Check sheet for the modelled part. Datum: model origin and axes. Units: mm. A direction names the side the tool comes from. Give positions to 0.01 mm unless a question says otherwise; leave off trailing zeros. Write each loop counter-clockwise with the first axis right and the second up, starting at its lowest first coordinate (ties: lowest second). Pieces come first, ordered by that corner, then holes. Notation, with made-up numbers: (72.5, 57) -> (83.5, 57) arc R21 cw to (83.5, 74) -> close; hole circle Ø6 at (67, 55). An arc over 180 degrees is marked (long way). Use a Markdown table: item, result. Add a question column.
1. Cross-section at A-A (x = -2.25). Enter the section's corners in (y, z).
2. Cross-section at B-B (y = -7.5). Enter the section's corners in (x, z).
3. Scan lines: probe 1 along Y at (x, z) = (0, 13); probe 2 along X at (y, z) = (-8.75, -19); probe 3 along X at (y, z) = (-1.5, 19.5). Record each from-to range of solid material in increasing order. Write a range as [from, to].
4. Release check for a two-part mould opening along Y. For faces 1 (the flat face through (0.754, 13.708, 0.35)), 2 (the flat face through (-12.804, 4.953, 0.35)), 3 (the flat face through (-5, 9, -25)), 4 (the flat face through (-3.537, -13.302, 0.35)) record: released by +Y, released by -Y, zero draft, split by the parting line, or undercut.
5. Set-up check for faces 5 (the cylindrical face through (-12.344, 1.969, 0.35)), 6 (the flat face through (7.474, 11.558, 0.35)), 7 (the cylindrical face through (8.85, 8.83, 0.35)): record each of +Z, -Z, +X, -X, +Y, -Y from which the full face is reachable in a straight line by a thin tool's end or side.
6. Gauge pin test, flat ends, axial feed: P1, Ø10, axis at y = 9, z = 4.5, coming from the -X side; P2, Ø3, axis at x = -12, z = 10.5, coming from the -Y side; P3, Ø1, axis at y = 8, z = 19.5, coming from the -X side. Record the tip position at first contact, or that the pin passes through.
from build123d import *

# Parameters (mm, degrees)
SKETCH1_R           = 10
BOSS_EXTRUDE1_DEPTH = 25


with BuildPart() as part:
    # Sketch1 → Boss-Extrude1 (new, symmetric)
    with BuildSketch(Plane.XY):
        with BuildLine():
            Line((-0.5, 14.991664351), (-1, 12.459935794))
            ThreePointArc((-1, 12.459935794), (-1.955430813, 12.346104257), (-2.899275393, 12.159120124))
            Line((-2.899275393, 12.159120124), (-4.1571508, 14.412428568))
            ThreePointArc((-4.1571508, 14.412428568), (-4.635254916, 14.265847744), (-5.108207316, 14.103411574))
            Line((-5.108207316, 14.103411574), (-4.801388426, 11.541086135))
            ThreePointArc((-4.801388426, 11.541086135), (-5.674881247, 11.137581552), (-6.51474951, 10.668085059))
            Line((-6.51474951, 10.668085059), (-8.407370715, 12.42240386))
            ThreePointArc((-8.407370715, 12.42240386), (-8.816778784, 12.135254916), (-9.21638771, 11.834618607))
            Line((-9.21638771, 11.834618607), (-8.132783499, 9.492514554))
            ThreePointArc((-8.132783499, 9.492514554), (-8.838834765, 8.838834765), (-9.492514554, 8.132783499))
            Line((-9.492514554, 8.132783499), (-11.834618607, 9.21638771))
            ThreePointArc((-11.834618607, 9.21638771), (-12.135254916, 8.816778784), (-12.42240386, 8.407370715))
            Line((-12.42240386, 8.407370715), (-10.668085059, 6.51474951))
            ThreePointArc((-10.668085059, 6.51474951), (-11.137581552, 5.674881247), (-11.541086135, 4.801388426))
            Line((-11.541086135, 4.801388426), (-14.103411574, 5.108207316))
            ThreePointArc((-14.103411574, 5.108207316), (-14.265847744, 4.635254916), (-14.412428568, 4.1571508))
            Line((-14.412428568, 4.1571508), (-12.159120124, 2.899275393))
            ThreePointArc((-12.159120124, 2.899275393), (-12.346104257, 1.955430813), (-12.459935794, 1))
            Line((-12.459935794, 1), (-14.991664351, 0.5))
            ThreePointArc((-14.991664351, 0.5), (-15, 0), (-14.991664351, -0.5))
            Line((-14.991664351, -0.5), (-12.459935794, -1))
            ThreePointArc((-12.459935794, -1), (-12.346104257, -1.955430813), (-12.159120124, -2.899275393))
            Line((-12.159120124, -2.899275393), (-14.412428568, -4.1571508))
            ThreePointArc((-14.412428568, -4.1571508), (-14.265847744, -4.635254916), (-14.103411574, -5.108207316))
            Line((-14.103411574, -5.108207316), (-11.541086135, -4.801388426))
            ThreePointArc((-11.541086135, -4.801388426), (-11.137581552, -5.674881247), (-10.668085059, -6.51474951))
            Line((-10.668085059, -6.51474951), (-12.42240386, -8.407370715))
            ThreePointArc((-12.42240386, -8.407370715), (-12.135254916, -8.816778784), (-11.834618607, -9.21638771))
            Line((-11.834618607, -9.21638771), (-9.492514554, -8.132783499))
            ThreePointArc((-9.492514554, -8.132783499), (-8.838834765, -8.838834765), (-8.132783499, -9.492514554))
            Line((-8.132783499, -9.492514554), (-9.21638771, -11.834618607))
            ThreePointArc((-9.21638771, -11.834618607), (-8.816778784, -12.135254916), (-8.407370715, -12.42240386))
            Line((-8.407370715, -12.42240386), (-6.51474951, -10.668085059))
            ThreePointArc((-6.51474951, -10.668085059), (-5.674881247, -11.137581552), (-4.801388426, -11.541086135))
            Line((-4.801388426, -11.541086135), (-5.108207316, -14.103411574))
            ThreePointArc((-5.108207316, -14.103411574), (-4.635254916, -14.265847744), (-4.1571508, -14.412428568))
            Line((-4.1571508, -14.412428568), (-2.899275393, -12.159120124))
            ThreePointArc((-2.899275393, -12.159120124), (-1.955430813, -12.346104257), (-1, -12.459935794))
            Line((-1, -12.459935794), (-0.5, -14.991664351))
            ThreePointArc((-0.5, -14.991664351), (0, -15), (0.5, -14.991664351))
            Line((0.5, -14.991664351), (1, -12.459935794))
            ThreePointArc((1, -12.459935794), (1.955430813, -12.346104257), (2.899275393, -12.159120124))
            Line((2.899275393, -12.159120124), (4.1571508, -14.412428568))
            ThreePointArc((4.1571508, -14.412428568), (4.635254916, -14.265847744), (5.108207316, -14.103411574))
            Line((5.108207316, -14.103411574), (4.801388426, -11.541086135))
            ThreePointArc((4.801388426, -11.541086135), (5.674881247, -11.137581552), (6.51474951, -10.668085059))
            Line((6.51474951, -10.668085059), (8.407370715, -12.42240386))
            ThreePointArc((8.407370715, -12.42240386), (8.816778784, -12.135254916), (9.21638771, -11.834618607))
            Line((9.21638771, -11.834618607), (8.132783499, -9.492514554))
            ThreePointArc((8.132783499, -9.492514554), (8.838834765, -8.838834765), (9.492514554, -8.132783499))
            Line((9.492514554, -8.132783499), (11.834618607, -9.21638771))
            ThreePointArc((11.834618607, -9.21638771), (12.135254916, -8.816778784), (12.42240386, -8.407370715))
            Line((12.42240386, -8.407370715), (10.668085059, -6.51474951))
            ThreePointArc((10.668085059, -6.51474951), (11.137581552, -5.674881247), (11.541086135, -4.801388426))
            Line((11.541086135, -4.801388426), (14.103411574, -5.108207316))
            ThreePointArc((14.103411574, -5.108207316), (14.265847744, -4.635254916), (14.412428568, -4.1571508))
            Line((14.412428568, -4.1571508), (12.159120124, -2.899275393))
            ThreePointArc((12.159120124, -2.899275393), (12.346104257, -1.955430813), (12.459935794, -1))
            Line((12.459935794, -1), (14.991664351, -0.5))
            ThreePointArc((14.991664351, -0.5), (15, 0), (14.991664351, 0.5))
            Line((14.991664351, 0.5), (12.459935794, 1))
            ThreePointArc((12.459935794, 1), (12.346104257, 1.955430813), (12.159120124, 2.899275393))
            Line((12.159120124, 2.899275393), (14.412428568, 4.1571508))
            ThreePointArc((14.412428568, 4.1571508), (14.265847744, 4.635254916), (14.103411574, 5.108207316))
            Line((14.103411574, 5.108207316), (11.541086135, 4.801388426))
            ThreePointArc((11.541086135, 4.801388426), (11.137581552, 5.674881247), (10.668085059, 6.51474951))
            Line((10.668085059, 6.51474951), (12.42240386, 8.407370715))
            ThreePointArc((12.42240386, 8.407370715), (12.135254916, 8.816778784), (11.834618607, 9.21638771))
            Line((11.834618607, 9.21638771), (9.492514554, 8.132783499))
            ThreePointArc((9.492514554, 8.132783499), (8.838834765, 8.838834765), (8.132783499, 9.492514554))
            Line((8.132783499, 9.492514554), (9.21638771, 11.834618607))
            ThreePointArc((9.21638771, 11.834618607), (8.816778784, 12.135254916), (8.407370715, 12.42240386))
            Line((8.407370715, 12.42240386), (6.51474951, 10.668085059))
            ThreePointArc((6.51474951, 10.668085059), (5.674881247, 11.137581552), (4.801388426, 11.541086135))
            Line((4.801388426, 11.541086135), (5.108207316, 14.103411574))
            ThreePointArc((5.108207316, 14.103411574), (4.635254916, 14.265847744), (4.1571508, 14.412428568))
            Line((4.1571508, 14.412428568), (2.899275393, 12.159120124))
            ThreePointArc((2.899275393, 12.159120124), (1.955430813, 12.346104257), (1, 12.459935794))
            Line((1, 12.459935794), (0.5, 14.991664351))
            ThreePointArc((0.5, 14.991664351), (0, 15), (-0.5, 14.991664351))
        make_face()
        Circle(SKETCH1_R, mode=Mode.SUBTRACT)
    extrude(amount=BOSS_EXTRUDE1_DEPTH, both=True)


solid = part.part
Worked answers:
| question | item | result |
|---|---|---|
| 1 | outline | (-12.3, -25) -> (-9.74, -25) -> (-9.74, 25) -> (-12.3, 25) -> close; (9.74, -25) -> (12.3, -25) -> (12.3, 25) -> (9.74, 25) -> close |
| 2 | outline | (-11.58, -25) -> (-6.61, -25) -> (-6.61, 25) -> (-11.58, 25) -> close; (6.61, -25) -> (11.58, -25) -> (11.58, 25) -> (6.61, 25) -> close |
| 3 | probe 1 | y = [-15, -10], [10, 15] |
| 3 | probe 2 | x = [-12.18, -10.83], [-8.93, -4.84], [4.84, 8.93], [10.83, 12.18] |
| 3 | probe 3 | x = [-12.41, -9.89], [9.89, 12.41] |
| 4 | face 1 | released by +Y |
| 4 | face 2 | undercut |
| 4 | face 3 | zero draft |
| 4 | face 4 | released by -Y |
| 5 | face 5 | +Z, -Z, -X |
| 5 | face 6 | +Z, -Z, +Y |
| 5 | face 7 | +Z, -Z |
| 6 | P1 | stops at x = -14.41 |
| 6 | P2 | stops at y = -9.22 |
| 6 | P3 | stops at x = -12.42 |
